```python
from build123d import *

# Parameters (mm, degrees)
SKETCH1_W           = 75
SKETCH1_H           = 45
SKETCH1_R           = 14
SKETCH1_R_2         = 1.6
BOSS_EXTRUDE1_DEPTH = 2.032
FILLET2_R           = 5
SKETCH2_R           = 1.6
CUT_EXTRUDE1_DEPTH  = 3.032
SKETCH5_W           = 21.294776471
SKETCH5_H           = 45
BOSS_EXTRUDE3_DEPTH = 2.032
FILLET3_R           = 5
SKETCH6_R           = 1.6
CUT_EXTRUDE2_DEPTH  = 3.032


with BuildPart() as part:
    # Sketch1 → Boss-Extrude1 (new body)
    with BuildSketch(Plane.XY):
        Rectangle(SKETCH1_W, SKETCH1_H)
        Circle(SKETCH1_R, mode=Mode.SUBTRACT)
        with Locations((-15.5, 15.5)):
            Circle(SKETCH1_R_2, mode=Mode.SUBTRACT)
        with Locations((15.5, 15.5)):
            Circle(SKETCH1_R_2, mode=Mode.SUBTRACT)
        with Locations((15.5, -15.5)):
            Circle(SKETCH1_R_2, mode=Mode.SUBTRACT)
        with Locations((-15.5, -15.5)):
            Circle(SKETCH1_R_2, mode=Mode.SUBTRACT)
    extrude(amount=BOSS_EXTRUDE1_DEPTH)

    # Fillet2
    fillet2_edges = [part.edges().sort_by_distance(p)[0] for p in [
        (37.5, -22.5, 1.016),
        (-37.5, -22.5, 1.016),
        (-37.5, 22.5, 1.016),
        (37.5, 22.5, 1.016),
    ]]
    fillet(fillet2_edges, radius=FILLET2_R)

    # Sketch2 → Cut-Extrude1 (cut, through all)
    with BuildSketch(Plane.XY.offset(2.032)):
        with Locations((-30, 0)):
            Circle(SKETCH2_R)
        with Locations((-30, 15)):
            Circle(SKETCH2_R)
        with Locations((-30, -15)):
            Circle(SKETCH2_R)
        with Locations((30, -15)):
            Circle(SKETCH2_R)
        with Locations((30, 15)):
            Circle(SKETCH2_R)
        with Locations((30, 0)):
            Circle(SKETCH2_R)
    extrude(amount=-CUT_EXTRUDE1_DEPTH, mode=Mode.SUBTRACT)

    # Sketch5 → Boss-Extrude3 (add)
    with BuildSketch(Plane.XY.offset(2.032)):
        with Locations((-43.032611765, 0)):
            Rectangle(SKETCH5_W, SKETCH5_H)
    extrude(amount=-BOSS_EXTRUDE3_DEPTH)

    # Fillet3
    fillet3_edges = [part.edges().sort_by_distance(p)[0] for p in [
        (-53.68, 22.5, 1.016),
        (-53.68, -22.5, 1.016),
    ]]
    fillet(fillet3_edges, radius=FILLET3_R)

    # Sketch6 → Cut-Extrude2 (cut, through all)
    with BuildSketch(Plane.XY.offset(2.032)):
        with Locations((-46.18, 15)):
            Circle(SKETCH6_R)
        with Locations((-46.18, 0)):
            Circle(SKETCH6_R)
        with Locations((-46.18, -15)):
            Circle(SKETCH6_R)
    extrude(amount=-CUT_EXTRUDE2_DEPTH, mode=Mode.SUBTRACT)


solid = part.part
```
Could you check a few things on this model? Use its own coordinates, in mm. Give positions to 0.01 mm unless a question says otherwise; leave off trailing zeros. Write each loop counter-clockwise with the first axis right and the second up, starting at its lowest first coordinate (ties: lowest second). Pieces come first, ordered by that corner, then holes. Notation, with made-up numbers: (25, 23.25) -> (64, 23.25) arc R11 ccw to (64, 30.25) -> close; hole circle Ø6 at (25.25, -4). An arc over 180 degrees is marked (long way). Write each question's results on one line, items separated by ' | '.
1. I need wall thicknesses on L1, parallel to Y at x = 30, z = 0.65; L2, parallel to Y at x = -15.5, z = 1.5; L3, parallel to Y at x = -16, z = 1.55. Which ranges of each line are inside material? Lowest first, please.
Check sheet entries:
L1: y = -22.5 to -16.6, -13.4 to -1.6, 1.6 to 13.4, 16.6 to 22.5 | L2: y = -22.5 to -17.1, -13.9 to 13.9, 17.1 to 22.5 | L3: y = -22.5 to -17.02, -13.98 to 13.98, 17.02 to 22.5
2. I want a section at B-B, the plane x = 15.5. Write out the boundary of the cut face in (y, z).
Check sheet entries:
outline: (-22.5, 0) -> (-17.1, 0) -> (-17.1, 2.03) -> (-22.5, 2.03) -> close; (-13.9, 0) -> (13.9, 0) -> (13.9, 2.03) -> (-13.9, 2.03) -> close; (17.1, 0) -> (22.5, 0) -> (22.5, 2.03) -> (17.1, 2.03) -> close
3. Will this pin go through, and if not, where does the flat tip stop? pin 1 Ø3 at (x, y) = (-15.5, 15.5) entering from -Z.
Check sheet entries:
pin 1: passes through
4. I want a section at A-A, the plane x = 30. Write out the boundary of the cut face in (y, z), then the cut area to 3 significant figures.
Check sheet entries:
outline: (-22.5, 0) -> (-16.6, 0) -> (-16.6, 2.03) -> (-22.5, 2.03) -> close; (-13.4, 0) -> (-1.6, 0) -> (-1.6, 2.03) -> (-13.4, 2.03) -> close; (1.6, 0) -> (13.4, 0) -> (13.4, 2.03) -> (1.6, 2.03) -> close; (16.6, 0) -> (22.5, 0) -> (22.5, 2.03) -> (16.6, 2.03) -> close | area: 71.9 mm²
5. If we mould it in two halves opening along X, with no side actions, what happens to faces 1 (the flat face through (-19, 0, 0)), 2 (the cylindrical face through (13.9, -15.43, 1)), 3 (the cylindrical face through (-52.25, -21, 1)), 4 (the flat face through (37.5, 0, 1))? For each: released by +X, released by -X, zero draft, split by the parting line, or undercut.
Check sheet entries:
face 1: zero draft | face 2: undercut | face 3: released by -X | face 4: released by +X
6. I want a section at C-C, the plane z = 1.05. Count the separate pieces of the cut face and the enclosed holes in it, then the cut area to 3 significant figures.
Check sheet entries:
separate pieces: 1 | enclosed holes: 14 | area: 3,360 mm²
7. I want a section at D-D, the plane y = 0. Write out the boundary of the cut face in (x, z).
Check sheet entries:
outline: (-53.68, 0) -> (-47.78, 0) -> (-47.78, 2.03) -> (-53.68, 2.03) -> close; (-44.58, 0) -> (-31.6, 0) -> (-31.6, 2.03) -> (-44.58, 2.03) -> close; (-28.4, 0) -> (-14, 0) -> (-14, 2.03) -> (-28.4, 2.03) -> close; (14, 0) -> (28.4, 0) -> (28.4, 2.03) -> (14, 2.03) -> close; (31.6, 0) -> (37.5, 0) -> (37.5, 2.03) -> (31.6, 2.03) -> close
